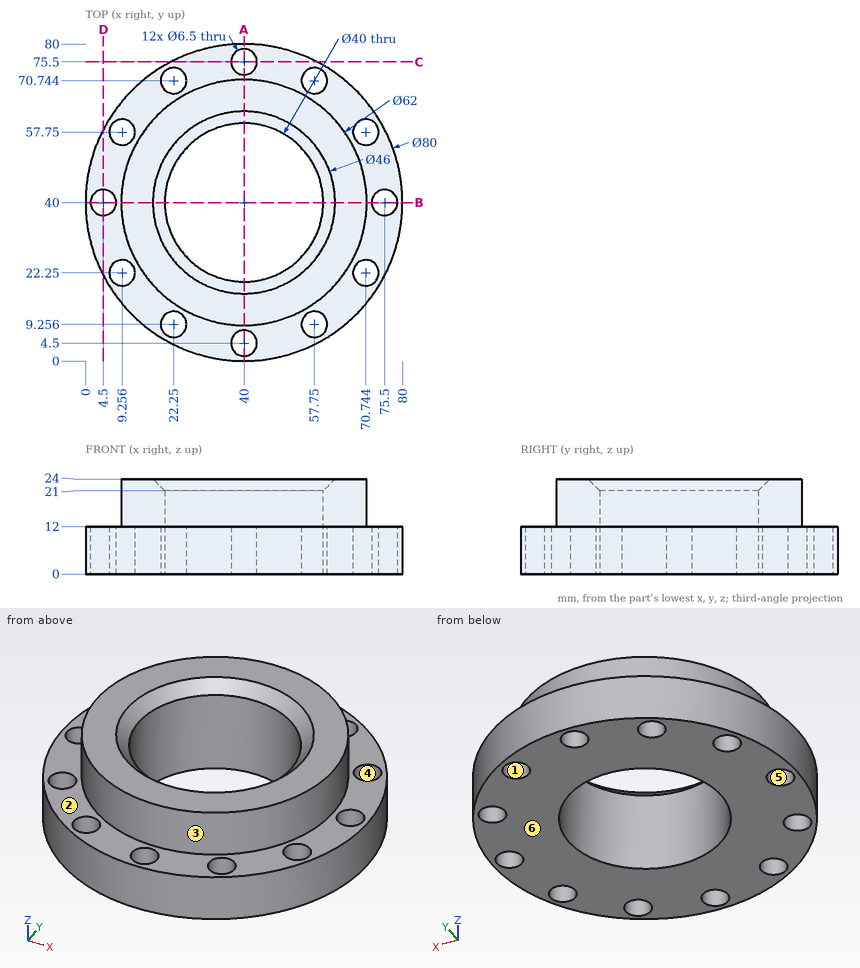
Verification items for this drawing (mm, ordinates from the low corner). A direction names the side the tool comes from. Coordinates: 2 decimals unless noted, no trailing zeros. Order: outer loops, then holes, each group sorted by start corner. A loop starts at its lowest first (then second) coordinate and runs counter-clockwise, first axis right, second up. Notation, with made-up numbers: M 15,-3 L 46,-3 A31 ccw 46,25 Z; hole C 8.25,-4.5 d3. An arc over 180 degrees is marked long. One line per item, written item: value. Start each with the question number.
Item 1: Thickness scan on probe 1 along Y at (x, z) = (57.75, 4.5); probe 2 along X at (y, z) = (9.5, 3); probe 3 along Y at (x, z) = (25, 10.5). Record the ranges inside material, lowest first.
Item 2: Sectioned sample at A-A on x = 40. Record the cut outline in (y, z), then the cut area to 3 significant figures.
Item 3: Access from +Z, -Z, +X, -X, +Y, -Y to the whole of each face (thin tool, end or side, straight path). Record for the marked faces 1 and 2.
Item 4: Depth check by flat-ended pin: P1, Ø4, axis at x = 29, y = 27, coming from the -Z side; P2, Ø10.5, axis at x = 57.75, y = 9.26, coming from the +Z side; P3, Ø5, axis at y = 30, z = 14, coming from the -X side; P4, Ø1.5, axis at y = 66.5, z = 14, coming from the +X side. Enter the tip coordinate at first touch or a pass-through.
Item 5: Mould release check, pull along Y, two halves, no side actions. Record for the marked faces 3, 4, 5 and 6: pulls with the +Y half, pulls with the -Y half, needs draft (parallel to the pull), parting line crosses it, or undercut.
Item 6: Sectioned sample at C-C on y = 75.5. Record the cut outline in (x, z), then the cut area to 3 significant figures.
Calculated:
1. probe 1: 4.15 to 6.01, 12.51 to 30.78, 49.22 to 67.49, 73.99 to 75.85
1. probe 2: 14.12 to 19.01, 25.49 to 54.51, 60.99 to 65.88
1. probe 3: 2.92 to 7.52, 10.99 to 26.77, 53.23 to 69.01, 72.48 to 77.08
2. outline: M 0,0 L 1.25,0 L 1.25,12 L 0,12 Z; M 7.75,0 L 20,0 L 20,21 L 17,24 L 9,24 L 9,12 L 7.75,12 Z; M 60,0 L 72.25,0 L 72.25,12 L 71,12 L 71,24 L 63,24 L 60,21 Z; M 78.75,0 L 80,0 L 80,12 L 78.75,12 Z
2. area: 579 mm^2
3. face 1: +Z, -Z
3. face 2: +Z
4. P1: through
4. P2: z = 24
4. P3: x = 0.91
4. P4: x = 57.26
5. face 3: parting line crosses it
5. face 4: undercut
5. face 5: undercut
5. face 6: needs draft
6. outline: M 21.57,0 L 36.75,0 L 36.75,12 L 21.57,12 Z; M 43.25,0 L 58.43,0 L 58.43,12 L 43.25,12 Z
6. area: 364 mm^2
